Autodesk Inventor part; units mm, degrees
ref_plane "YZ Plane" through (0, 0, 0) normal (1, 0, 0) x (0, 1, 0)
ref_plane "XZ Plane" through (0, 0, 0) normal (0, 1, 0) x (-1, 0, 0)
ref_plane "XY Plane" through (0, 0, 0) normal (0, 0, 1) x (1, 0, 0)
sketch "Esboço1" plane through (0, 0, 0) normal (1, 0, 0) x (0, 1, 0)
  line L0 (-504, 129) -> (504, 129)
  line L1 (504, 129) -> (504, -129)
  line L2 (504, -129) -> (-504, -129)
  line L3 (-504, -129) -> (-504, 129)
  line L4 (-504, 129) -> (504, -129) construction
  line L5 (504, 129) -> (-504, -129) construction
  point P0 (0, 0)
  dimension "d0" = 1008
  dimension "d1" = 258
extrude "Extrusão1" add sketch "Esboço1" along normal mid plane 4
sketch "Esboço2" plane through (2, 0, 0) normal (1, 0, 0) x (0, 0, -1)
  line L0 (-133, 378) -> (-125, 378)
  line L1 (-125, 378) -> (-125, 126)
  line L2 (-125, 126) -> (-133, 126)
  line L3 (-133, 126) -> (-133, 378)
  line L4 (-129, 504) -> (-129, -504)
  line L5 (-133, 378) -> (-125, 126) construction
  line L6 (-125, 378) -> (-133, 126) construction
  line L7 (129, 504) -> (-129, 504)
  line L8 (-133, -126) -> (-125, -126)
  line L9 (-125, -126) -> (-125, -378)
  line L10 (-125, -378) -> (-133, -378)
  line L11 (-133, -378) -> (-133, -126)
  line L12 (-133, -126) -> (-125, -378) construction
  line L13 (-125, -126) -> (-133, -378) construction
  line L14 (-129, -504) -> (129, -504)
  line L15 (125, 378) -> (133, 378)
  line L16 (133, 378) -> (133, 126)
  line L17 (133, 126) -> (125, 126)
  line L18 (125, 126) -> (125, 378)
  line L19 (129, -504) -> (129, 504)
  line L20 (125, 378) -> (133, 126) construction
  line L21 (133, 378) -> (125, 126) construction
  line L22 (125, -126) -> (133, -126)
  line L23 (133, -126) -> (133, -378)
  line L24 (133, -378) -> (125, -378)
  line L25 (125, -378) -> (125, -126)
  line L26 (125, -126) -> (133, -378) construction
  line L27 (133, -126) -> (125, -378) construction
  point P0 (0, 0)
  point P1 (-129, 252)
  point P2 (-129, -252)
  point P3 (129, 252)
  point P4 (129, -252)
  dimension "d4" = 8
  dimension "d5" = 252
  dimension "d6" = 126
  dimension "d7" = 8
  dimension "d8" = 252
  dimension "d9" = 252
  dimension "d10" = 126
  dimension "d11" = 126
  dimension "d12" = 252
  dimension "d13" = 8
  dimension "d14" = 252
  dimension "d15" = 8
  dimension "d16" = 252
  dimension "d17" = 126
extrude "Extrusão2" cut sketch "Esboço2" along normal through all both and the other way through all contours L0 L4 L2 L3 | L0 L1 L2 L4 | L8 L9 L10 L4 | L4 L10 L11 L8 | L19 L17 L18 L15 | L15 L16 L17 L19 | L22 L23 L24 L19 | L19 L24 L25 L22
sketch "Esboço3" plane through (2, 0, 0) normal (1, 0, 0) x (0, 0, -1)
  line L0 (-41.5, 500) -> (41.5, 500)
  line L1 (41.5, 500) -> (41.5, 508)
  line L2 (41.5, 508) -> (-41.5, 508)
  line L3 (-41.5, 508) -> (-41.5, 500)
  line L4 (129, 504) -> (-129, 504)
  line L5 (-41.5, 500) -> (41.5, 508) construction
  line L6 (41.5, 500) -> (-41.5, 508) construction
  line L7 (-41.5, -500) -> (41.5, -500)
  line L8 (41.5, -500) -> (41.5, -508)
  line L9 (41.5, -508) -> (-41.5, -508)
  line L10 (-41.5, -508) -> (-41.5, -500)
  line L11 (-129, -504) -> (129, -504)
  line L12 (-41.5, -500) -> (41.5, -508) construction
  line L13 (41.5, -500) -> (-41.5, -508) construction
  point P0 (0, 0)
  point P1 (0, 504)
  point P2 (0, -504)
  dimension "d20" = 83
  dimension "d21" = 8
  dimension "d22" = 83
  dimension "d23" = 8
extrude "Extrusão3" cut sketch "Esboço3" along normal through all both and the other way through all
sketch "Esboço4" plane through (2, 0, 0) normal (1, 0, 0) x (0, 0, -1)
  line L0 (41.5, 500) -> (-41.5, 500)
  line L1 (-41.5, 438) -> (-37.5, 438)
  line L2 (-37.5, 438) -> (-37.5, 378)
  line L3 (-37.5, 378) -> (-41.5, 378)
  line L4 (-41.5, 378) -> (-41.5, 438)
  point P0 (0, 0)
  dimension "d26" = 62
  dimension "d27" = 4
  dimension "d28" = 60
extrude "Extrusão4" cut sketch "Esboço4" against normal through all
pattern_linear "Padrão retangular1" count 2 spacing 80 along (0, 0, -1) count 2 spacing 818 along (0, -1, 0) of "Extrusão4"
properties part number "FUNDO"
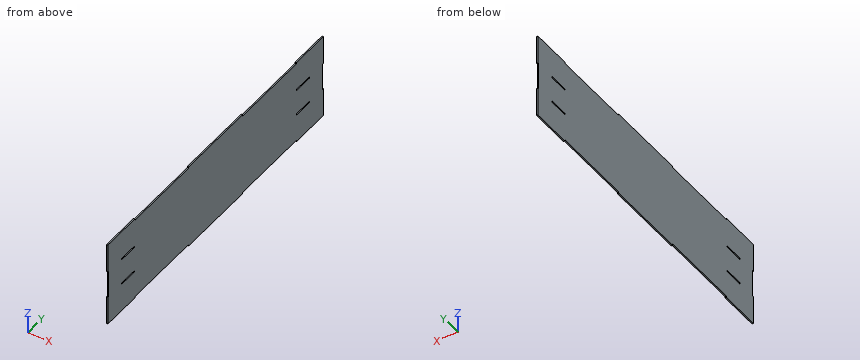
The model under review builds one solid part; all positions refer to its coordinate system, in mm. Round coordinates to 2 decimals unless told otherwise and drop trailing zeros. Order: outer loops, then holes, each group sorted by start corner. A loop starts at its lowest first (then second) coordinate and runs counter-clockwise, first axis right, second up. Notation, with made-up numbers: (-27.5, -37.75) -> (15.5, -37.75) arc R8 ccw to (15.5, -24.75) -> close; hole circle Ø3 at (-18.75, 62). An arc over 180 degrees is marked (long way). Use CSV: the item, a comma, the result in double quotes. Start each with the question number.
(1) Consider section B-B on y = -339.5. Write out the cut boundary in (x, z).
(2) Consider section A-A on x = -0.1. State how many separate pieces and enclosed holes the cut face has, and give its area (3 significant figures).
(3) Insertion check: pin 1 (1.2 mm diameter, centred on x = -0.5, z = 40, fed in from +Y); pin 2 (1.2 mm diameter, centred on x = 0, y = 248, fed in from +Z); pin 3 (1.2 mm diameter, centred on x = 0, z = 39, fed in from -Y). Each pin has a flat end and moves straight along its axis. Give the tip position at first contact, or say it passes through.
(4) Wall thickness on probe 1 along Z at (x, y) = (-0.95, 423); probe 2 along Y at (x, z) = (0.5, -40); probe 3 along Z at (x, y) = (-0.3, -335.5): over which ranges is each line inside the solid? List them lowest first. Write a range as from..to.
Responses:
1,outline,"(-2, -125) -> (2, -125) -> (2, 125) -> (-2, 125) -> close"
2,separate pieces,"1"
2,enclosed holes,"4"
2,area,"254,000 mm²"
3,pin 1,"y = 500"
3,pin 2,"z = 125"
3,pin 3,"y = -500"
4,probe 1,"-129..-42.5, -38.5..37.5, 41.5..129"
4,probe 2,"-500..-440, -380..378, 438..500"
4,probe 3,"-125..125"
